Build history of the part. All positions in model axes, mm. Face numbers are marked on the shaded views. A direction names the side the tool comes from. Coordinates: 2 decimals unless noted, no trailing zeros. Order: outer loops, then holes, each group sorted by start corner. A loop starts at its lowest first (then second) coordinate and runs counter-clockwise, first axis right, second up. Notation, with made-up numbers: (86.5, 82) -> (139.5, 82) arc R28 ccw to (139.5, 114) -> close; hole circle Ø4 at (28.5, 76). An arc over 180 degrees is marked (long way). Write each question's results on one line, items separated by ' | '.
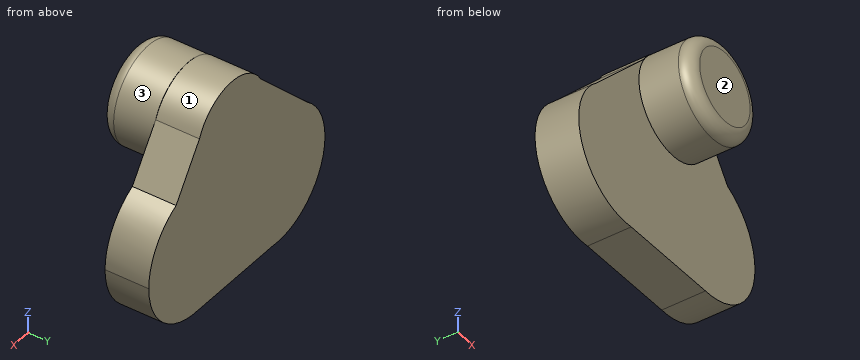
from build123d import *

# Parameters (mm, degrees)
F1_DEPTH = 25.654
F2_R     = 28.4407370428
F3_DEPTH = 30.48
F4_R     = 7.3585229381


with BuildPart() as f1:
    # F0 (on Front) → F1 (new body)
    with BuildSketch(Plane.XZ):
        with BuildLine():
            ThreePointArc((-21.5344435526, 2.0731437555), (-4.8204991058, 5.3895527458), (7.0882450204, 17.5771005261))
            ThreePointArc((7.0882450204, 17.5771005261), (-8.8670748097, 12.8601538234), (-21.5344435526, 2.0731437555))
        make_face()
        with BuildLine():
            ThreePointArc((7.9605099877, 41.948206774), (9.6731432739, 36.4370915007), (10.2517769659, 30.6950807571))
            ThreePointArc((10.2517769659, 30.6950807571), (9.4497176108, 23.9480566036), (7.0882450204, 17.5771005261))
            ThreePointArc((7.0882450204, 17.5771005261), (17.5408909724, 17.0287274663), (27.4955300755, 13.793966155))
            Line((27.4955300755, 13.793966155), (7.9605099877, 41.948206774))
        make_face()
        with BuildLine():
            ThreePointArc((-23.7264411014, -43.725716795), (-36.04104655, -57.2814370335), (-53.1818165378, -63.731325619))
            Line((-53.1818165378, -63.731325619), (8.938396841, -62.4778672324))
            ThreePointArc((8.938396841, -62.4778672324), (-9.7326904365, -57.1755765902), (-23.7264411014, -43.725716795))
        make_face()
        with BuildLine():
            ThreePointArc((-18.9324777024, -24.9800812453), (-20.5427988057, -13.8821683024), (-25.2409413599, -3.6996213576))
            ThreePointArc((-25.2409413599, -3.6996213576), (-29.8392434552, -23.915311506), (-23.7264411014, -43.725716795))
            ThreePointArc((-23.7264411014, -43.725716795), (-20.1499486388, -34.6545442437), (-18.9324777024, -24.9800812453))
        make_face()
        with BuildLine():
            ThreePointArc((27.4955300755, 13.793966155), (17.5408909724, 17.0287274663), (7.0882450204, 17.5771005261))
            ThreePointArc((7.0882450204, 17.5771005261), (-4.8204991058, 5.3895527458), (-21.5344435526, 2.0731437555))
            ThreePointArc((-21.5344435526, 2.0731437555), (-23.5113697235, -0.7338297985), (-25.2409413599, -3.6996213576))
            ThreePointArc((-25.2409413599, -3.6996213576), (-20.5427988057, -13.8821683024), (-18.9324777024, -24.9800812453))
            ThreePointArc((-18.9324777024, -24.9800812453), (-20.1499486388, -34.6545442437), (-23.7264411014, -43.725716795))
            ThreePointArc((-23.7264411014, -43.725716795), (-9.7326904365, -57.1755765902), (8.938396841, -62.4778672324))
            ThreePointArc((8.938396841, -62.4778672324), (38.12540726, -51.2074452523), (50.331310131, -22.3991144449))
            ThreePointArc((50.331310131, -22.3991144449), (44.1452046519, -1.0016149762), (27.4955300755, 13.793966155))
        make_face()
        with BuildLine():
            ThreePointArc((7.0882450204, 17.5771005261), (9.4497176108, 23.9480566036), (10.2517769659, 30.6950807571))
            ThreePointArc((10.2517769659, 30.6950807571), (9.6731432739, 36.4370915007), (7.9605099877, 41.948206774))
            ThreePointArc((7.9605099877, 41.948206774), (-16.4945513192, 59.4026144185), (-43.1654741186, 45.5690231721))
            ThreePointArc((-43.1654741186, 45.5690231721), (-44.2964170336, 17.8799643072), (-21.5344435526, 2.0731437555))
            ThreePointArc((-21.5344435526, 2.0731437555), (-8.8670748097, 12.8601538234), (7.0882450204, 17.5771005261))
        make_face()
        with BuildLine():
            ThreePointArc((-21.5344435526, 2.0731437555), (-44.2964170336, 17.8799643072), (-43.1654741186, 45.5690231721))
            Line((-43.1654741186, 45.5690231721), (-82.2833511654, 5.5814185032))
            ThreePointArc((-82.2833511654, 5.5814185032), (-51.7089264452, 13.5602395088), (-25.2409413599, -3.6996213576))
            ThreePointArc((-25.2409413599, -3.6996213576), (-23.5113697235, -0.7338297985), (-21.5344435526, 2.0731437555))
        make_face()
        with BuildLine():
            ThreePointArc((-25.2409413599, -3.6996213576), (-51.7089264452, 13.5602395088), (-82.2833511654, 5.5814185032))
            ThreePointArc((-82.2833511654, 5.5814185032), (-93.9821658408, -40.0960598334), (-53.1818165378, -63.731325619))
            ThreePointArc((-53.1818165378, -63.731325619), (-36.04104655, -57.2814370335), (-23.7264411014, -43.725716795))
            ThreePointArc((-23.7264411014, -43.725716795), (-29.8392434552, -23.915311506), (-25.2409413599, -3.6996213576))
        make_face()
    extrude(amount=-F1_DEPTH)

    # F2 (on Front) → F3 (join)
    with BuildSketch(Plane.XZ):
        with Locations((-18.2904135436, 31.1521012336)):
            Circle(F2_R)
    extrude(amount=F3_DEPTH)

    # F4
    f4_edges = [f1.edges().sort_by_distance(p)[0] for p in [
        (-46.731151, -30.48, 31.152101),
    ]]
    fillet(f4_edges, radius=F4_R)


solid = f1.part
Item 1: Drill centre lines: line 1 (Y direction, x = 31.5, z = -54.5); line 2 (Z direction, x = -55, y = 9); line 3 (X direction, y = -5.5, z = 26). Where is each one in solid material? Low to high. Write a range as from..to.
Answer:
line 1: y = 0..25.65 | line 2: z = -63.91..33.47 | line 3: x = -46.26..9.68
Item 2: Slice it at D-D, the plane y = -17. List the corners of the cut face in (x, z), and give its area (3 significant figures).
Answer:
outline: circle Ø56.88 at (-18.29, 31.15) | area: 2,540 mm^2
Item 3: Slice it at B-B, the plane z = -46.5. List the corners of the cut face in (x, y).
Answer:
outline: (-90.56, 0) -> (42.28, 0) -> (42.28, 25.65) -> (-90.56, 25.65) -> close
Item 4: Pin check, flat tips, straight feed: pin 1 (1.5 mm diameter, centred on x = -51, y = 6.5, fed in from +Z); pin 2 (12 mm diameter, centred on x = 23, y = 17.5, fed in from -Z); pin 3 (12 mm diameter, centred on y = -16, z = 19, fed in from +X). Stop position of each tip, or through.
Answer:
pin 1: stops at z = 38.33 | pin 2: stops at z = -61.92 | pin 3: stops at x = 9.48
Item 5: Slice it at A-A, the plane y = 10. List the corners of the cut face in (x, z), and give its area (3 significant figures).
Answer:
outline: (-82.28, 5.58) arc R39.05 ccw to (-53.18, -63.73) -> (8.94, -62.48) arc R40.1 ccw to (27.5, 13.79) -> (7.96, 41.95) arc R28.78 ccw to (-43.17, 45.57) -> close | area: 13,000 mm^2
Item 6: Tool access for the marked faces 1, 2 and 3: list every direction of +Z, -Z, +X, -X, +Y, -Y with a clear straight run to the whole face (end or side of a thin tool).
Answer:
face 1: +Z, +Y | face 2: +Z, -Z, +X, -X, -Y | face 3: -Y
Item 7: Slice it at C-C, the plane x = -87. List the corners of the cut face in (y, z), and give its area (3 significant figures).
Answer:
outline: (0, -51.1) -> (25.65, -51.1) -> (25.65, 1.14) -> (0, 1.14) -> close | area: 1,340 mm^2
